Input: part model. Units: mm. Frame: model coordinates. Coordinates: 2 decimals unless noted, no trailing zeros. Use one line per item in the form item = value. Start each with the question number.
1) Section query A-A on z = 2. Count the separate pieces of the cut face and the enclosed holes in it, then the cut area to 3 significant figures.
2) Pin query (flat end, axial travel): pin 1 (3 mm diameter, centred on x = 17.5, y = 39, fed in from -Z). Return the tip coordinate at first contact, or that it passes through.
3) Ray query, line 1 along X through (y, z) = (5.5, 0.5); line 2 along X through (y, z) = (43.5, 4.75); line 3 along Y through (x, z) = (76.5, 2.75). Return the intervals inside material, ascending.
Autodesk Inventor part; units mm, degrees
ref_plane "YZ Plane" through (0, 0, 0) normal (1, 0, 0) x (0, 1, 0)
ref_plane "XZ Plane" through (0, 0, 0) normal (0, 1, 0) x (-1, 0, 0)
ref_plane "XY Plane" through (0, 0, 0) normal (0, 0, 1) x (1, 0, 0)
sketch "Sketch1" plane through (0, 0, 0) normal (0, 0, 1) x (1, 0, 0)
  line L0 (0, 0) -> (82.55, 0)
  line L1 (82.55, 0) -> (82.55, 50.8)
  line L2 (82.55, 50.8) -> (0, 50.8)
  line L3 (0, 50.8) -> (0, 0)
  dimension "d0" = 50.8
  dimension "d1" = 82.55
extrude "Extrusion1" add sketch "Sketch1" along normal blind 6.35
fillet "Fillet1" radius 3.175 4 edges at (82.55, 50.8, 3.175) (82.55, 0, 3.175) (0, 0, 3.175) (0, 50.8, 3.175)
sketch "Sketch2" plane through (0, 0, 6.35) normal (0, 0, 1) x (1, 0, 0)
  line L0 (5.2705, 45.4025) -> (77.2795, 45.4025) construction
  line L1 (77.2795, 45.4025) -> (77.2795, 5.3975) construction
  line L2 (77.2795, 5.3975) -> (5.2705, 5.3975) construction
  line L3 (5.2705, 5.3975) -> (5.2705, 45.4025) construction
  line L4 (0, 47.625) -> (0, 3.175) construction
  line L5 (79.375, 50.8) -> (3.175, 50.8) construction
  point P0 (0, 0)
  point P1 (5.2705, 25.4)
  point P2 (0, 25.4)
  point P3 (41.275, 45.4025)
  point P4 (41.275, 50.8)
  dimension "d5" = 72.009
  dimension "d6" = 40.005
hole "Hole1" at (5.2705, 45.4025, 6.35) at (77.2795, 45.4025, 6.35) at (77.2795, 5.3975, 6.35) at (5.2705, 5.3975, 6.35) direction (0, 0, -1) diameter 5.1054 end through all
properties part number "LL-001" material "ABS Plastic"
Answers below:
q1.separate_pieces = 1
q1.enclosed_holes = 4
q1.area = 4,100 mm^2
q2.pin_1 = 0
q3.line_1 = 0 to 2.72, 7.82 to 74.73, 79.83 to 82.55
q3.line_2 = 0 to 3.57, 6.97 to 75.58, 78.98 to 82.55
q3.line_3 = 0 to 2.97, 7.83 to 42.97, 47.83 to 50.8
